Work out the finished part from the listing and answer in its coordinate system (mm). Face numbers are marked on the shaded views. A direction names the side the tool comes from. Coordinates: 2 decimals unless noted, no trailing zeros. Order: outer loops, then holes, each group sorted by start corner. A loop starts at its lowest first (then second) coordinate and runs counter-clockwise, first axis right, second up. Notation, with made-up numbers: M -20.5,39 L 33.5,39 A27 cw 33.5,56 Z; hole C 39,-8 d10. An arc over 180 degrees is marked long. Answer in a Markdown table with one row per item. Add a question column.
Item 1: The part is cut by section C-C (y = 30). State how many separate pieces and enclosed holes the cut face has, then the cut area to 3 significant figures.
Item 2: The part is cut by section A-A (x = -63). Write down the section's boundary in (y, z) (3 decimals).
Item 3: Which of the six approach directions +Z, -Z, +X, -X, +Y, -Y give full straight-line access (tool end or side, diameter ignored) to the marked faces 4, 5, 6 and 7?
Item 4: The mould has two halves that part along X. Classify the marked faces 1, 2 and 3: released by +X, released by -X, zero draft, split by the parting line, or undercut.
Item 5: Flat-ended cylindrical pins translate along their axes: pin 1 Ø1 at (y, z) = (18, 63.5) entering from +X (3 decimals); pin 2 Ø12 at (y, z) = (15, 16) entering from -X (3 decimals); pin 3 Ø2 at (y, z) = (17.5, 57.5) entering from -X (3 decimals); pin 4 Ø18.5 at (x, z) = (-115.89, 23.81) entering from -Y. Find the tip coordinate at first contact, or state that the pin passes through.
Item 6: The part is cut by section D-D (x = -44). Write down the section's boundary in (y, z).
Item 7: Consider line 1 (Y direction, x = -107, z = 61); line 2 (X direction, y = 19, z = 57.5) (3 decimals); line 3 (Z direction, x = -10, y = 32) (3 decimals). Determine where each line is inside the solid, lowest interval first. Write a range as from..to.
Item 8: The part is cut by section B-B (z = 21.5). Write down the section's boundary in (x, y) (3 decimals), then the cut area to 3 significant figures.
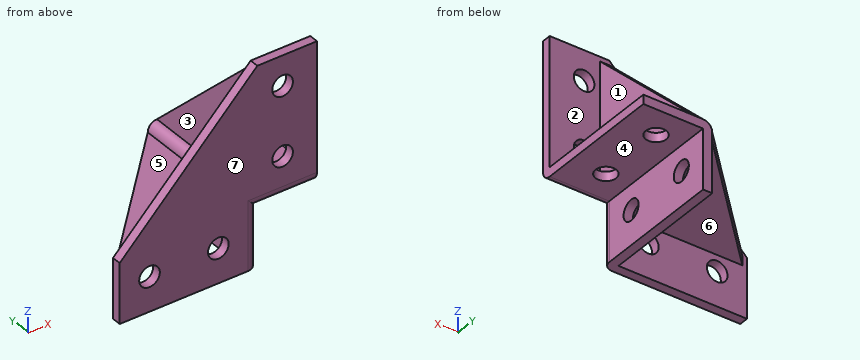
from build123d import *

# Parameters (mm, degrees)
BASE_PLATE_DEPTH      = 6.35
SKETCH2_W             = 6.35
SKETCH2_H             = 47.625
UPPER_LEAF_DEPTH      = 88.9
LOFT1_START           = 34.925
LOFT1_DEPTH           = 6.35
SKETCH10_W            = 7.14375
SKETCH10_H            = 47.62505
SKETCH10_AT_POINT_2_W = 7.14375
SKETCH10_AT_POINT_2_H = 47.62505
SKETCH10_AT_POINT_3_W = 7.14375
SKETCH10_AT_POINT_3_H = 47.62505
SKETCH10_AT_POINT_4_W = 7.14375
SKETCH10_AT_POINT_4_H = 47.62505
FILLET1_R             = 6.35


# Read off the part's stored shape, not the designer's step: Loft1, Mirror1
with BuildPart() as part:
    # Sketch1 → Base Plate (new body)
    with BuildSketch(Plane(origin=(0, 0, 0), x_dir=(1, 0, 0), z_dir=(0, 1, 0))):
        Polygon((-136.525, 0), (-41.275, 0), (-41.275, -41.275), (0, -41.275), (0, -136.525), (-41.275, -136.525), (-136.525, -41.275), align=None)
    extrude(amount=BASE_PLATE_DEPTH)

    # Sketch2 → Upper Leaf (add)
    with BuildSketch(Plane(origin=(0, 6.35, 0), x_dir=(1, 0, 0), z_dir=(0, 1, 0))):
        with Locations((-44.45, -23.8125)):
            Rectangle(SKETCH2_W, SKETCH2_H)
    extrude(amount=UPPER_LEAF_DEPTH)

    # Loft1 outline → Loft1 (add)
    with BuildSketch(Plane.XY.offset(LOFT1_START)):
        Polygon((-47.625, 6.35), (-47.625, 95.25), (-133.35, 6.35), align=None)
    extrude(amount=LOFT1_DEPTH)

    # Sketch10 → 9/16 (0.5625) Diameter Hole1 (revolve, cut)
    with BuildSketch(Plane(origin=(-47.625, 74.6125, 23.8125), x_dir=(0, 0, 1), z_dir=(0, 1, 0))):
        with Locations((3.571875, 23.812525)):
            Rectangle(SKETCH10_W, SKETCH10_H)
    revolve(axis=Axis((-53.975, 74.6125, 23.8125), (1, 0, 0)), mode=Mode.SUBTRACT)

    # Sketch10 at point 2 (carried to point 2, square into its face) → 9/16 (0.5625) Diameter Hole1 at 2 (revolve, cut)
    with BuildSketch(Plane(origin=(-47.625, 26.9875, 23.8125), x_dir=(0, 0, 1), z_dir=(0, 1, 0))):
        with Locations((3.571875, 23.812525)):
            Rectangle(SKETCH10_AT_POINT_2_W, SKETCH10_AT_POINT_2_H)
    revolve(axis=Axis((-53.975, 26.9875, 23.8125), (1, 0, 0)), mode=Mode.SUBTRACT)

    # Sketch10 at point 3 (carried to point 3, square into its face) → 9/16 (0.5625) Diameter Hole1 at 3 (revolve, cut)
    with BuildSketch(Plane(origin=(-68.2625, 6.35, 23.8125), x_dir=(0, 0, 1), z_dir=(1, 0, 0))):
        with Locations((3.571875, 23.812525)):
            Rectangle(SKETCH10_AT_POINT_3_W, SKETCH10_AT_POINT_3_H)
    revolve(axis=Axis((-68.2625, 12.7, 23.8125), (0, -1, 0)), mode=Mode.SUBTRACT)

    # Sketch10 at point 4 (carried to point 4, square into its face) → 9/16 (0.5625) Diameter Hole1 at 4 (revolve, cut)
    with BuildSketch(Plane(origin=(-115.8875, 6.35, 23.8125), x_dir=(0, 0, 1), z_dir=(1, 0, 0))):
        with Locations((3.571875, 23.812525)):
            Rectangle(SKETCH10_AT_POINT_4_W, SKETCH10_AT_POINT_4_H)
    revolve(axis=Axis((-115.8875, 12.7, 23.8125), (0, -1, 0)), mode=Mode.SUBTRACT)

    # Mirror1
    split(bisect_by=Plane(origin=(0, 0, 0), x_dir=(-0.7071067811865476, 0, 0.7071067811865476), z_dir=(0.7071067811865477, 0, 0.7071067811865475)), keep=Keep.BOTTOM)

    # Mirror1 2: part across plane


with BuildPart() as part_1:
    add(part.part)
    add(part.part.mirror(Plane(origin=(0, 0, 0), x_dir=(-0.7071067811865476, 0, 0.7071067811865476), z_dir=(0.7071067811865477, 0, 0.7071067811865475))))

    # Fillet1
    fillet1_edges = [part_1.edges().sort_by_distance(p)[0] for p in [
        (-41.275, 0, 20.6375),
        (-20.6375, 0, 41.275),
        (-47.625, 50.8, 47.625),
    ]]
    fillet(fillet1_edges, radius=FILLET1_R - 0.0001)  # a hair under: the kernel refuses the full size


solid = part_1.part
Reply:
| question | item | result |
|---|---|---|
| 1 | separate pieces | 3 |
| 1 | enclosed holes | 0 |
| 1 | area | 1,190 mm2 |
| 2 | outline | M 0,0 L 6.35,0 L 6.35,18.981 L 0,18.981 Z; M 0,28.644 L 6.35,28.644 L 6.35,34.925 L 79.306,34.925 L 79.306,41.275 L 6.35,41.275 L 6.35,114.8 L 0,114.8 Z |
| 3 | face 4 | -Z, +X, +Y, -Y |
| 3 | face 5 | +Z, -X, +Y |
| 3 | face 6 | -Z, -X, +Y |
| 3 | face 7 | +Z, -Z, +X, -X, -Y |
| 4 | face 1 | released by +X |
| 4 | face 2 | zero draft |
| 4 | face 3 | released by -X |
| 5 | pin 1 | stops at x = -34.925 |
| 5 | pin 2 | stops at x = -47.625 |
| 5 | pin 3 | stops at x = -41.275 |
| 5 | pin 4 | stops at y = 0 |
| 6 | outline | M 0,47.62 A6.35 ccw 1.14,44 L 1.14,0 L 95.25,0 L 95.25,47.01 L 6.35,47.01 L 6.35,133.8 L 0,133.8 Z; hole C 26.99,23.81 d14.29; hole C 74.61,23.81 d14.29 |
| 7 | line 1 | y = 0..6.35 |
| 7 | line 2 | x = -41.275..-34.925 |
| 7 | line 3 | z = 41.275..47.625 |
| 8 | outline | M -136.525,0 L -122.647,0 L -122.647,6.35 L -136.525,6.35 Z; M -109.128,0 L -75.022,0 L -75.022,6.35 L -109.128,6.35 Z; M -61.503,0 L -47.625,0 A6.35 ccw -41.275,6.35 L -41.275,20.228 L -47.625,20.228 L -47.625,6.35 L -61.503,6.35 Z; M -47.625,33.747 L -41.275,33.747 L -41.275,67.853 L -47.625,67.853 Z; M -47.625,81.372 L -41.275,81.372 L -41.275,95.25 L -47.625,95.25 Z |
| 8 | area | 817 mm2 |
